from build123d import *

# Parameters (mm, degrees)
F0_W      = 1500
F0_H      = 730
F0_W_2    = 1398.4
F0_H_2    = 628.4
F1_DEPTH  = 50.8
F3_DEPTH  = 50.8
F4_W      = 50.8
F4_H      = 25.4
F5_DEPTH  = 101.6
F6_R      = 12.5
F7_DEPTH  = 25
F8_R      = 12.5
F9_DEPTH  = 25
F10_W     = 50.8
F10_H     = 50.8
F11_DEPTH = 923.8


with BuildPart() as f1:
    # F0 (on Right) → F1 (new body)
    with BuildSketch(Plane.YZ):
        with Locations((-750, 365)):
            Rectangle(F0_W, F0_H)
        with Locations((-750, 365)):
            Rectangle(F0_W_2, F0_H_2, mode=Mode.SUBTRACT)
    extrude(amount=F1_DEPTH)

    # F2 (on face) → F3 (join, through all)
    with BuildSketch(Plane(origin=(0, 0, 0), x_dir=(0, -1, 0), z_dir=(-1, 0, 0))):
        Polygon((759.037996, 396.728377), (117.181979, 679.2), (50.8, 679.2), (50.8, 637.002018), (677.904086, 361.022508), (50.8, 85.042998), (50.8, 50.8), (99.105988, 50.8), (740.962004, 333.271623), (1382.818021, 50.8), (1449.2, 50.8), (1449.2, 92.997982), (822.095914, 368.977492), (1449.2, 644.957002), (1449.2, 679.2), (1400.894012, 679.2), align=None)
    extrude(amount=-F3_DEPTH)

    # F4 (on face) → F5 (join)
    with BuildSketch(Plane(origin=(0, 0, 0), x_dir=(-1, 0, 0), z_dir=(0, 1, 0))):
        with Locations((-25.4, 717.3)):
            Rectangle(F4_W, F4_H)
        with Locations((-25.4, 12.7)):
            Rectangle(F4_W, F4_H)
    extrude(amount=F5_DEPTH)

    # F6 (on face) → F7 (join)
    with BuildSketch(Plane.XY.offset(730)):
        with Locations((25.4, 76.2)):
            Circle(F6_R)
    extrude(amount=F7_DEPTH)

    # F8 (on face) → F9 (join)
    with BuildSketch(Plane(origin=(0, 0, 0), x_dir=(1, 0, 0), z_dir=(0, 0, -1))):
        with Locations((25.4, -76.2)):
            Circle(F8_R)
    extrude(amount=F9_DEPTH)

    # F10 (on face) → F11 (join)
    with BuildSketch(Plane.YZ.offset(50.8)):
        with Locations((-1474.6, 704.6)):
            Rectangle(F10_W, F10_H)
        with Locations((-1474.6, 25.4)):
            Rectangle(F10_W, F10_H)
    extrude(amount=F11_DEPTH)


solid = f1.part
For this review, take the finished solid that the model builds, in its own axes (mm). A direction names the side the tool comes from. Give positions to 0.01 mm unless a question says otherwise; leave off trailing zeros. Order: outer loops, then holes, each group sorted by start corner. A loop starts at its lowest first (then second) coordinate and runs counter-clockwise, first axis right, second up. Notation, with made-up numbers: (25, 58) - (81, 58) arc R18 cw to (81, 79) - close; hole circle Ø2 at (-12.5, -40). An arc over 180 degrees is marked (long way). Answer as a JSON object with one key per item and string values. Group by question number.
Item 1: Take a section at B-B on z = 461.5. Give the boundary of the cut face in (x, y).
Item 2: Draft analysis for pull direction Y (two halves, no side actions). For faces 5 (the flat face through (506, -1475, 50.8)), 6 (the flat face through (25, -1449.2, 365)), 7 (the flat face through (25, 0, 360)), 8 (the flat face through (25, -750, 50.8)), state which applies: pulls with the +Y half, pulls with the -Y half, needs draft (parallel to the pull), parting line crosses it, or undercut.
Item 3: Take a section at C-C on y = -164. Give the boundary of the cut face in (x, z).
Item 4: Wall thickness on line 1 along Y through (x, z) = (122, 37); line 2 along X through (y, z) = (-223, 147): over which ranges is each line inside the solid? List them lowest first.
Item 5: Clearance check with flat-ended pins moving along their axes: pin 1 Ø4 at (y, z) = (-1188, 529) entering from +X; pin 2 Ø15 at (x, z) = (37, 465.5) entering from +Y. State where each tip first meets the part, or that it passes through.
Item 6: Take a section at A-A on x = 454.5. Give the boundary of the cut face in (y, z).
Item 7: Machinability: for faces 1 (the flat face through (506, -1475, 679.2)), 2 (the flat face through (506, -1449.2, 704)), 3 (the flat face through (26, 50, 704.6)), 4 (the flat face through (25.044, -368.742, 224.965)), which of the approach directions +Z, -Z, +X, -X, +Y, -Y give a long, thin tool a straight path to every point of the face, cutting with its end or side? Answer none if there is none.
Reported:
{
 "1": {"outline": "(0, -1500) - (50.8, -1500) - (50.8, -1449.2) - (0, -1449.2) - close; (0, -1032.33) - (50.8, -1032.33) - (50.8, -906.22) - (0, -906.22) - close; (0, -611.86) - (50.8, -611.86) - (50.8, -449.59) - (0, -449.59) - close; (0, -50.8) - (50.8, -50.8) - (50.8, 0) - (0, 0) - close"},
 "2": {"face 5": "needs draft", "face 6": "undercut", "face 7": "pulls with the +Y half", "face 8": "undercut"},
 "3": {"outline": "(0, 0) - (50.8, 0) - (50.8, 50.8) - (0, 50.8) - close; (0, 79.36) - (50.8, 79.36) - (50.8, 134.86) - (0, 134.86) - close; (0, 587.18) - (50.8, 587.18) - (50.8, 658.6) - (0, 658.6) - close; (0, 679.2) - (50.8, 679.2) - (50.8, 730) - (0, 730) - close"},
 "4": {"line 1": "-1500 to -1449.2", "line 2": "0 to 50.8"},
 "5": {"pin 1": "x = 50.8", "pin 2": "y = 0"},
 "6": {"outline": "(-1500, 0) - (-1449.2, 0) - (-1449.2, 50.8) - (-1500, 50.8) - close; (-1500, 679.2) - (-1449.2, 679.2) - (-1449.2, 730) - (-1500, 730) - close"},
 "7": {"face 1": "+X, +Y, -Y", "face 2": "+Z, -Z, +X, +Y", "face 3": "+X, -X, +Y", "face 4": "+X, -X"}
}
